Build history of the part. All positions in model axes, mm. Give positions to 0.01 mm unless a question says otherwise; leave off trailing zeros. Write each loop counter-clockwise with the first axis right and the second up, starting at its lowest first coordinate (ties: lowest second). Pieces come first, ordered by that corner, then holes. Notation, with made-up numbers: M 30,40 L 50,40 A10 ccw 50,46 Z; hole C 37.25,86 d7. An arc over 180 degrees is marked long. Return JSON: item names as keys, results as strings. Group by question number.
Q1. Band-saw the part on A-A, the plane x = -16.5. Give the cut face in (y, z), then the cut area to 4 significant figures.
Q2. Flat gauge pins, fed straight in: pin 1 Ø2 at (x, y) = (16.5, 2.5) entering from +Z; pin 2 Ø1.5 at (x, y) = (78, 3.5) entering from -Z; pin 3 Ø10 at (x, z) = (-24, 68.5) entering from -Y; pin 4 Ø3 at (x, y) = (-85.5, 1.5) entering from +Z. Where does each tip first touch, or does it go through?
Q3. Wall check: probe 1 along X at (y, z) = (1, -4); probe 2 along Z at (x, y) = (90.8, 2.5) (3 decimals); probe 3 along Z at (x, y) = (89.35, 2.5) (3 decimals). Give the ranges that are in metal, low to high.
from build123d import *

# Parameters (mm, degrees)
SKETCH1_W               = 185
SKETCH1_H               = 313
BASE_DEPTH              = 5
SKETCH2_W               = 20
SKETCH2_H               = 5
BOSS_EXTRUDE2_DEPTH     = 5
LPATTERN1_COUNT         = 2
LPATTERN1_PITCH         = 55
LPATTERN1_COL_COUNT     = 2
LPATTERN1_COL_PITCH     = 55
SKETCH3_W               = 4
SKETCH3_H               = 20
CUT_EXTRUDE1_DEPTH      = 187.181363192
LPATTERN2_COUNT         = 3
LPATTERN2_PITCH         = 55
LPATTERN2_COL_COUNT     = 3
LPATTERN2_COL_PITCH     = 55
FILLET1_R               = 10
MIRROR1_COPY_1_SKETCH_W = 20
MIRROR1_COPY_1_SKETCH_H = 5
MIRROR1_COPY_1_DEPTH    = 5
MIRROR1_COPY_2_SKETCH_W = 20
MIRROR1_COPY_2_SKETCH_H = 5
MIRROR1_COPY_2_DEPTH    = 5
CUT_EXTRUDE4_DEPTH      = 187.181363192
LPATTERN5_COUNT         = 4
LPATTERN5_PITCH         = 84.333333333
CUT_EXTRUDE5_DEPTH      = 187.181363192


with BuildPart() as part:
    # Sketch1 → Base (new body)
    with BuildSketch(Plane(origin=(0, 0, 0), x_dir=(1, 0, 0), z_dir=(0, 1, 0))):
        Rectangle(SKETCH1_W, SKETCH1_H)
    extrude(amount=BASE_DEPTH)

    # Sketch2 → Boss-Extrude2 (add)
    with BuildSketch(Plane(origin=(0, 5, 0), x_dir=(1, 0, 0), z_dir=(0, 1, 0))):
        with Locations((0, -159)):
            Rectangle(SKETCH2_W, SKETCH2_H)
    boss_extrude2 = extrude(amount=-BOSS_EXTRUDE2_DEPTH)

    # LPattern1: Boss-Extrude2 ×2
    with Locations(*[(-i * LPATTERN1_PITCH, 0, 0) for i in range(1, LPATTERN1_COUNT)]):
        add(boss_extrude2)

    # LPattern1 col: Boss-Extrude2 ×2
    with Locations(*[(i * LPATTERN1_COL_PITCH, 0, 0) for i in range(1, LPATTERN1_COL_COUNT)]):
        add(boss_extrude2)

    # Sketch3 → Cut-Extrude1 (cut, through all)
    with BuildSketch(Plane(origin=(0, 5, 0), x_dir=(1, 0, 0), z_dir=(0, 1, 0))):
        with Locations((-85.5, 0)):
            Rectangle(SKETCH3_W, SKETCH3_H)
    cut_extrude1 = extrude(amount=-CUT_EXTRUDE1_DEPTH, mode=Mode.SUBTRACT)

    # LPattern2: Cut-Extrude1 ×3
    with Locations(*[(0, 0, -i * LPATTERN2_PITCH) for i in range(1, LPATTERN2_COUNT)]):
        add(cut_extrude1, mode=Mode.SUBTRACT)

    # LPattern2 col: Cut-Extrude1 ×3
    with Locations(*[(0, 0, i * LPATTERN2_COL_PITCH) for i in range(1, LPATTERN2_COL_COUNT)]):
        add(cut_extrude1, mode=Mode.SUBTRACT)

    # Fillet1
    fillet1_edges = [part.edges().sort_by_distance(p)[0] for p in [
        (-92.5, 2.5, -156.5),
        (92.5, 2.5, -156.5),
        (92.5, 2.5, 156.5),
        (-92.5, 2.5, 156.5),
    ]]
    fillet(fillet1_edges, radius=FILLET1_R)

    # Mirror1: Boss-Extrude2 across plane
    add(boss_extrude2.mirror(Plane.XY))

    # Mirror1 copy 1 sketch → Mirror1 copy 1 (add)
    with BuildSketch(Plane(origin=(-55, 5, 0), x_dir=(1, 0, 0), z_dir=(0, 1, 0))):
        with Locations((0, 159)):
            Rectangle(MIRROR1_COPY_1_SKETCH_W, MIRROR1_COPY_1_SKETCH_H)
    extrude(amount=-MIRROR1_COPY_1_DEPTH)

    # Mirror1 copy 2 sketch → Mirror1 copy 2 (add)
    with BuildSketch(Plane(origin=(55, 5, 0), x_dir=(1, 0, 0), z_dir=(0, 1, 0))):
        with Locations((0, 159)):
            Rectangle(MIRROR1_COPY_2_SKETCH_W, MIRROR1_COPY_2_SKETCH_H)
    extrude(amount=-MIRROR1_COPY_2_DEPTH)

    # Sketch5 → Cut-Extrude4 (cut, through all)
    with BuildSketch(Plane(origin=(0, 5, 0), x_dir=(1, 0, 0), z_dir=(0, 1, 0))):
        Polygon((-63.667363032, 141.40999982), (-70.5, 141.40999982), (-70.5, 136.502092421), (-70.5, 82.79999982), (-60.23, 82.79999982), (-60.23, 88.26099982), (-49.211989258, 88.26099982), (-49.211989258, 101.65899982), (-62.23, 101.65899982), (-62.23, 105.27899982), (-46.895, 105.27899982), (-46.895, 125.28099982), (-60.23, 125.28099982), (-60.23, 133.244848009), (-60.23, 141.40999982), align=None)
    extrude(amount=-CUT_EXTRUDE4_DEPTH, mode=Mode.SUBTRACT)

    # Sketch8 → Tap Drill for M2.5x0.45 Tap1 (revolve, cut)
    with BuildSketch(Plane(origin=(92.5, 2.5, -126.5), x_dir=(0, 0, -1), z_dir=(0, 1, 0))):
        Polygon((0, 0), (0, 5.615882135), (1.025, 5), (1.025, 0), align=None)
    tap_drill_for_m2_5x0_45_tap1 = revolve(axis=Axis((98.85, 2.5, -126.5), (-1, 0, 0)), mode=Mode.SUBTRACT)

    # LPattern5: Tap Drill for M2.5x0.45 Tap1 ×4
    with Locations(*[(0, 0, i * LPATTERN5_PITCH) for i in range(1, LPATTERN5_COUNT)]):
        add(tap_drill_for_m2_5x0_45_tap1, mode=Mode.SUBTRACT)

    # Sketch9 → Cut-Extrude5 (cut, through all)
    with BuildSketch(Plane(origin=(0, 0, 0), x_dir=(-1, 0, 0), z_dir=(0, -1, 0))):
        Polygon((46.895, 105.27899982), (46.895, 88.26099982), (49.211989258, 88.26099982), (49.211989258, 101.65899982), (62.23, 101.65899982), (62.23, 105.27899982), (49.211989258, 105.27899982), align=None)
    extrude(amount=-CUT_EXTRUDE5_DEPTH, mode=Mode.SUBTRACT)


solid = part.part
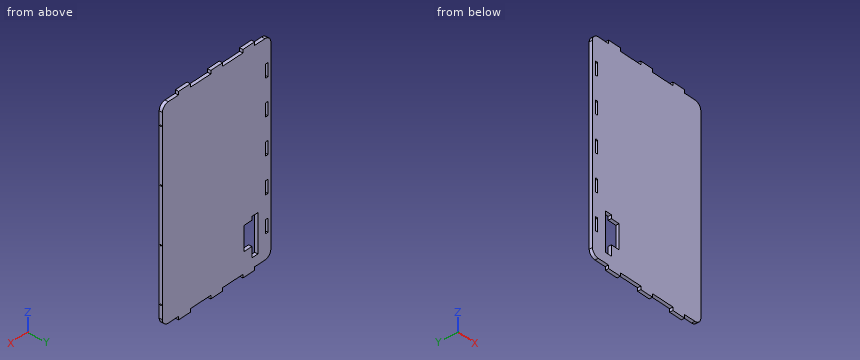
From the geometry:
{
 "1": {"outline": "M 0,-156.5 L 5,-156.5 L 5,156.5 L 0,156.5 Z", "area": "1,565 mm^2"},
 "2": {"pin 1": "stops at z = 156.5", "pin 2": "stops at z = -156.5", "pin 3": "stops at y = 0", "pin 4": "stops at z = 156.39"},
 "3": {"probe 1": "x = -92.5 to -87.5, -83.5 to 92.5", "probe 2": "z = -152.078 to -127.525, -125.475 to -43.192, -41.142 to 41.142, 43.192 to 125.475, 127.525 to 152.078", "probe 3": "z = -153.785 to -127.525, -125.475 to -43.192, -41.142 to 41.142, 43.192 to 125.475, 127.525 to 153.785"}
}
